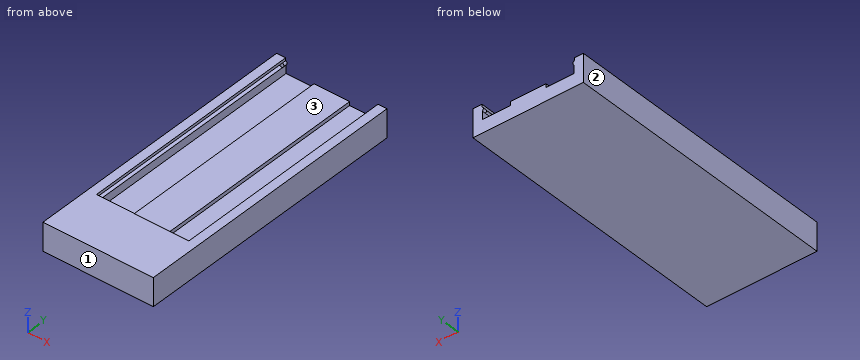
from build123d import *

# Parameters (mm, degrees)
BOSS_EXTRUDE1_DEPTH = 381
SKETCH4_R           = 3.175
BOSS_EXTRUDE2_DEPTH = 5.08
BOSS_EXTRUDE3_START = -5.08
SKETCH5_R           = 3.175
BOSS_EXTRUDE3_DEPTH = 5.08
SCALE1_SCALE        = 0.7
SKETCH8_W           = 105
SKETCH8_H           = 26.67
BOSS_EXTRUDE6_DEPTH = 50.8


with BuildPart() as part:
    # Sketch3 → Boss-Extrude1 (new body)
    with BuildSketch(Plane(origin=(0, 0, 0), x_dir=(1, 0, 0), z_dir=(0, 1, 0))):
        with BuildLine():
            Line((0, 0), (0, 38.1))
            Line((0, 38.1), (150, 38.1))
            Line((150, 38.1), (150, 0))
            Line((150, 0), (137.808, 0))
            Line((137.808, 0), (137.808, 3.81))
            ThreePointArc((137.808, 3.81), (142.319844489, 6.978228189), (137.3, 9.257607897))
            Line((137.3, 9.257607897), (137.3, 20.32))
            Line((137.3, 20.32), (99.2, 20.32))
            Line((99.2, 20.32), (99.2, 15.24))
            Line((99.2, 15.24), (50.8, 15.24))
            Line((50.8, 15.24), (50.8, 20.32))
            Line((50.8, 20.32), (12.7, 20.32))
            Line((12.7, 20.32), (12.7, 9.257607897))
            ThreePointArc((12.7, 9.257607897), (7.680155511, 6.978228189), (12.192, 3.81))
            Line((12.192, 3.81), (12.192, 0))
            Line((12.192, 0), (0, 0))
        make_face()
    extrude(amount=BOSS_EXTRUDE1_DEPTH)

    # Sketch4 → Boss-Extrude2 (add)
    with BuildSketch(Plane(origin=(0, 0, 0), x_dir=(1, 0, 0), z_dir=(0, 1, 0))):
        with Locations((10.841440118, 6.683432269)):
            Circle(SKETCH4_R)
        with Locations((139.158559882, 6.683432269)):
            Circle(SKETCH4_R)
    extrude(amount=BOSS_EXTRUDE2_DEPTH)

    # Sketch5 → Boss-Extrude3 (add)
    with BuildSketch(Plane(origin=(0, 381, 0), x_dir=(1, 0, 0), z_dir=(0, 1, 0)).offset(BOSS_EXTRUDE3_START)):
        with Locations((139.158559882, 6.683432269)):
            Circle(SKETCH5_R)
        with Locations((10.841440118, 6.683432269)):
            Circle(SKETCH5_R)
    extrude(amount=BOSS_EXTRUDE3_DEPTH)


with BuildPart() as part_1:
    # Scale1: scaled about (75, 190.5, -25.842389862)
    add(part.part.scale(SCALE1_SCALE).moved(Location((22.5, 57.15, -7.752716959))))

    # Sketch8 → Boss-Extrude6 (add)
    with BuildSketch(Plane.XZ.offset(-57.15)):
        with Locations((75, -21.087716959)):
            Rectangle(SKETCH8_W, SKETCH8_H)
    extrude(amount=-BOSS_EXTRUDE6_DEPTH)


solid = part_1.part
Here's how the part is built. I have some questions about the finished solid (model axes, mm). Face numbers are marked on the shaded views. Give positions to 0.01 mm unless a question says otherwise; leave off trailing zeros. Loops run counter-clockwise (first coordinate to the right, second up) from the corner with the lowest first, then second, coordinate; pieces in that order, holes last. Notation, with made-up numbers: (44.5, -12) -> (71.5, -12) arc R27 ccw to (71.5, 4) -> close; hole circle Ø6 at (78.5, -8). An arc over 180 degrees is marked (long way). Answer as a JSON object with one key per item and string values. Group by question number.
Item 1: I need wall thicknesses on L1, parallel to X at y = 300, z = -21; L2, parallel to X at y = 162, z = -17; L3, parallel to Y at x = 58, z = -16. Which ranges of each line are inside material? Lowest first, please.
Item 2: Imagine slicing it at C-C on x = 72.5. Write out the boundary of the cut face in (y, z), then the cut area to 3 significant figures.
Item 3: Imagine slicing it at A-A on y = 139. Write out the boundary of the cut face in (x, z) (1 decimal).
Item 4: Will these pins go through, and if not, where does the flat tip stop? pin 1 (10 mm diameter, centred on x = 77.5, y = 175, fed in from +Z); pin 2 (21.5 mm diameter, centred on x = 43.5, y = 181.5, fed in from +Z); pin 3 (4.5 mm diameter, centred on x = 59, z = -15, fed in from +Y).
Item 5: Thinking about a two-plate mould opening in X: for the marked faces 1, 2 and 3, which applies, pulls with the +X half, pulls with the -X half, needs draft (parallel to the pull), parting line crosses it, or undercut?
Item 6: Imagine slicing it at B-B on x = 51.5. Write out the boundary of the cut face in (y, z), then the cut area to 3 significant figures.
Answer list:
{
 "1": {"L1": "x = 22.5 to 31.39, 58.06 to 91.94, 118.61 to 127.5", "L2": "x = 22.5 to 31.39, 118.61 to 127.5", "L3": "y = 57.15 to 107.95"},
 "2": {"outline": "(57.15, -34.42) -> (323.85, -34.42) -> (323.85, -18.42) -> (107.95, -18.42) -> (107.95, -7.75) -> (57.15, -7.75) -> close", "area": "4,810 mm2"},
 "3": {"outline": "(22.5, -34.4) -> (127.5, -34.4) -> (127.5, -7.8) -> (119, -7.8) -> (119, -10.4) arc R2.2 cw (long way) to (118.6, -14.2) -> (118.6, -22) -> (91.9, -22) -> (91.9, -18.4) -> (58.1, -18.4) -> (58.1, -22) -> (31.4, -22) -> (31.4, -14.2) arc R2.2 cw (long way) to (31, -10.4) -> (31, -7.8) -> (22.5, -7.8) -> close"},
 "4": {"pin 1": "stops at z = -18.42", "pin 2": "stops at z = -21.98", "pin 3": "stops at y = 107.95"},
 "5": {"face 1": "needs draft", "face 2": "pulls with the -X half", "face 3": "undercut"},
 "6": {"outline": "(57.15, -34.42) -> (323.85, -34.42) -> (323.85, -21.98) -> (107.95, -21.98) -> (107.95, -7.75) -> (57.15, -7.75) -> close", "area": "4,040 mm2"}
}
